The model under review builds one solid part; all positions refer to its coordinate system, in mm. A direction names the side the tool comes from. Coordinates: 2 decimals unless noted, no trailing zeros. Order: outer loops, then holes, each group sorted by start corner. A loop starts at its lowest first (then second) coordinate and runs counter-clockwise, first axis right, second up.
```python
from build123d import *

# Parameters (mm, degrees)
F0_R            = 74
F1_DEPTH        = 25
F2_R            = 60
F3_DEPTH        = 3
F4_D            = 17
F6_D            = 8.5
F6_COPIES_COUNT = 6
F8_D            = 12.7
F8_CBORE_D      = 19.1
F8_CBORE_DEPTH  = 13.1
F8_COPIES_COUNT = 6


# Not quite as in the source:
# - a pattern or mirror of a feature is missing from the dataset's text; its kind, count and spacing are read off the source's solid


with BuildPart() as f1:
    # F0 (on Top) → F1 (new body)
    with BuildSketch(Plane.XY):
        Circle(F0_R)
    extrude(amount=F1_DEPTH)

    # F2 (on face) → F3 (join)
    with BuildSketch(Plane.XY.offset(25)):
        Circle(F2_R)
    extrude(amount=F3_DEPTH)

    # F4 (through all)
    with Locations(Plane(origin=(0, 0, 0), x_dir=(1, 0, 0), z_dir=(0, 0, -1))):
        with Locations((0, 0)):
            Hole(F4_D / 2)

    # F6 (through all)
    with Locations(Plane.XY.offset(25)):
        with Locations((0, 66)):
            f6 = Hole(F6_D / 2)

    # F6_copies: F6 ×6 about axis
    f6_copies_axis = Axis((0, 0, 0), (0, 0, 1))
    for i in range(1, F6_COPIES_COUNT):
        add(f6.rotate(f6_copies_axis, i * 360 / F6_COPIES_COUNT), mode=Mode.SUBTRACT)

    # F8 (through all)
    with Locations(Plane.XY.offset(28)):
        with Locations((0, 45)):
            f8 = CounterBoreHole(F8_D / 2, F8_CBORE_D / 2, F8_CBORE_DEPTH)

    # F8_copies: F8 ×6 about axis
    f8_copies_axis = Axis((0, 0, 0), (0, 0, 1))
    for i in range(1, F8_COPIES_COUNT):
        add(f8.rotate(f8_copies_axis, i * 360 / F8_COPIES_COUNT), mode=Mode.SUBTRACT)


solid = f1.part
```
(1) Wall thickness on probe 1 along X at (y, z) = (-28, 15.5); probe 2 along Y at (x, z) = (4.5, 9.75); probe 3 along Y at (x, z) = (41.5, 17.5): over which ranges is each line inside the solid? List them lowest first.
A:
probe 1: x = -68.5 to -46.78, -31.16 to 31.16, 46.78 to 68.5
probe 2: y = -73.86 to -49.48, -40.52 to -7.21, 7.21 to 40.52, 49.48 to 73.86
probe 3: y = -61.27 to -31.71, -13.29 to 13.29, 31.71 to 61.27
(2) We need section D-D, the plane z = 1.75. Count the separate pieces of the cut face and the enclosed holes in it, and give its area (3 significant figures).
A:
separate pieces: 1
enclosed holes: 13
area: 15,900 mm2
(3) We need section B-B, the plane x = -57.5. Write out the cut boundary in (y, z).
A:
outline: (-46.58, 0) - (-37.24, 0) - (-37.24, 25) - (-46.58, 25) - close; (-28.76, 0) - (28.76, 0) - (28.76, 25) - (17.14, 25) - (17.14, 28) - (-17.14, 28) - (-17.14, 25) - (-28.76, 25) - close; (37.24, 0) - (46.58, 0) - (46.58, 25) - (37.24, 25) - close
(4) Draft analysis for pull direction Y (two halves, no side actions). For faces 3 (the face through (-1, -12, 28)), 4 (the face through (2.07, -35.677, 21.542)), 5 (the face through (-16.04, -72.24, 12.32)), state which applies: released by +Y, released by -Y, zero draft, split by the parting line, or undercut.
A:
face 3: zero draft
face 4: undercut
face 5: split by the parting line
(5) Machinability: for faces 1 (the face through (-1.38, -38.8, 7.35)), 2 (the face through (-34.57, -17.66, 14.9)), which of the approach directions +Z, -Z, +X, -X, +Y, -Y give a long, thin tool a straight path to every point of the face, cutting with its end or side? Answer none if there is none.
A:
face 1: +Z, -Z
face 2: +Z
(6) We need section C-C, the plane y = 22.5. Write out the cut boundary in (x, z).
A:
outline: (-70.5, 0) - (-45.32, 0) - (-45.32, 14.9) - (-48.52, 14.9) - (-48.52, 28) - (-55.62, 28) - (-55.62, 25) - (-70.5, 25) - close; (-32.62, 0) - (32.62, 0) - (32.62, 14.9) - (29.42, 14.9) - (29.42, 28) - (-29.42, 28) - (-29.42, 14.9) - (-32.62, 14.9) - close; (45.32, 0) - (70.5, 0) - (70.5, 25) - (55.62, 25) - (55.62, 28) - (48.52, 28) - (48.52, 14.9) - (45.32, 14.9) - close
(7) For pin 1 Ø2 at (x, y) = (-42, 15) entering from -Z; pin 2 Ø5 at (x, z) = (-36.5, 19.5) entering from +Y; pin 3 Ø12 at (y, z) = (23, 24) entering from +X; pin 4 Ø5.5 at (x, y) = (3.5, -41) entering from +Z, all flat-tipped, find the tip position at first contact; note any pin that passes through.
A:
pin 1: stops at z = 0
pin 2: stops at y = 65.73
pin 3: stops at x = 72.02
pin 4: stops at z = 14.9
(8) We need section A-A, the plane y = 0. Write out the cut boundary in (x, z).
A:
outline: (-74, 0) - (-8.5, 0) - (-8.5, 28) - (-60, 28) - (-60, 25) - (-74, 25) - close; (8.5, 0) - (74, 0) - (74, 25) - (60, 25) - (60, 28) - (8.5, 28) - close
